Read the model definition and answer for the solid it produces. Units are mm, in the model's axes. A direction names the side the tool comes from. Round coordinates to 2 decimals unless told otherwise and drop trailing zeros. Order: outer loops, then holes, each group sorted by start corner. A loop starts at its lowest first (then second) coordinate and runs counter-clockwise, first axis right, second up. Notation, with made-up numbers: (33.5, 41) - (40.5, 41) arc R23 cw to (40.5, 65) - close; hole circle Ø6 at (-7.5, -23). An arc over 180 degrees is marked (long way). Put each result on its own line as item: value. Start each with the question number.
Q1. Which of the six approach directions +Z, -Z, +X, -X, +Y, -Y give full straight-line access (tool end or side, diameter ignored) to faces 4 (the face through (15.875, -3, -24)), 5 (the face through (3, -6.35, -14))?
Q2. Section A-A on y = -2 is taken. State how many separate pieces and enclosed holes the cut face has, then the cut area to 3 significant figures.
Q3. Section C-C on z = -6 is taken. Give the vertices of the cut face in (x, y) (3 decimals).
Q4. For a pull along Z with two mould halves and no side action, classify faces 1 (the face through (22, -3, -62.454)), 2 (the face through (30, -3, -46.579)), 3 (the face through (-0.42, -3.13, -56.03)) as pulls with the +Z half, pulls with the -Z half, needs draft (parallel to the pull), parting line crosses it, or undercut.
Q5. Section B-B on z = -28 is taken. Give the vertices of the cut face in (x, y) (3 decimals), then the cut area to 3 significant figures.
Q6. Find the intervals of material crossed by line 1 along Z through (x, y) = (2, -2.75); line 2 along Z through (x, y) = (-2, -2.5); line 3 along Z through (x, y) = (21, -2), in increasing order. Write a range as from..to.
Q7. Each of these flat-tipped pins is pushed along its axis until it touches: pin 1 Ø7.5 at (x, z) = (0.27, -52.93) entering from +Y; pin 2 Ø1 at (y, z) = (-4, -41) entering from +X (3 decimals); pin 3 Ø1.9 at (x, y) = (31, -3.5) entering from +Z; pin 4 Ø5 at (x, z) = (0, 0) entering from -Y. Where does it stop, or does it pass through?
from build123d import *

# Parameters (mm, degrees)
F0_R     = 3.175
F1_DEPTH = 6.35


# Not quite as in the source:
# - the program builds the solid bodies; features that only make, move or delete a surface that nothing else refers to are left out


with BuildPart() as f1:
    # F0 (on Front) → F1 (new body)
    with BuildSketch(Plane.XZ):
        with BuildLine():
            ThreePointArc((15.7504882737, 1.984375), (10.5003255158, 11.90625), (0, 15.875))
            ThreePointArc((0, 15.875), (-10.500325544, 11.9062499751), (-15.7504882831, 1.9843749253))
            ThreePointArc((-15.7504882831, 1.9843749253), (-15.875, -5.44e-08), (-15.7504882695, -1.9843750333))
            ThreePointArc((-15.7504882695, -1.9843750333), (0.9941387534, -15.8438414893), (15.875, 0))
            ThreePointArc((15.875, 0), (15.8440389276, 0.9909871135), (15.7512764776, 1.9781087752))
            ThreePointArc((15.7512764776, 1.9781087752), (15.7508826872, 1.9812419268), (15.7504882737, 1.984375))
        make_face()
        with BuildLine():
            ThreePointArc((0, 3.175), (2.2450640303, 2.2450640303), (3.175, 0))
            ThreePointArc((3.175, 0), (-2.2450640303, -2.2450640303), (0, 3.175))
        make_face(mode=Mode.SUBTRACT)
        with BuildLine():
            ThreePointArc((-15.7504882831, 1.9843749253), (-10.500325544, 11.9062499751), (0, 15.875))
            Line((0, 15.875), (0, 41.275))
            ThreePointArc((0, 41.275), (-7.14375, 44.4998046905), (-9.4502929642, 51.990625))
            Line((-9.4502929642, 51.990625), (-15.7504882831, 1.9843749253))
        make_face()
        with BuildLine():
            Line((0, 41.275), (0, 15.875))
            ThreePointArc((0, 15.875), (10.5003255158, 11.90625), (15.7504882737, 1.984375))
            Line((15.7504882737, 1.984375), (9.4502929642, 51.990625))
            ThreePointArc((9.4502929642, 51.990625), (9.5063048942, 51.396483242), (9.525, 50.8))
            ThreePointArc((9.525, 50.8), (6.7351920908, 44.0648079092), (0, 41.275))
        make_face()
        with BuildLine():
            ThreePointArc((-15.7504882695, -1.9843750333), (-15.875, -5.44e-08), (-15.7504882831, 1.9843749253))
            Line((-15.7504882831, 1.9843749253), (-16.0004960241, 0))
            Line((-16.0004960241, 0), (-15.7504882695, -1.9843750333))
        make_face()
        with BuildLine():
            ThreePointArc((-9.4502929642, 51.990625), (-7.14375, 44.4998046905), (0, 41.275))
            ThreePointArc((0, 41.275), (6.7351920908, 44.0648079092), (9.525, 50.8))
            ThreePointArc((9.525, 50.8), (9.5063048942, 51.396483242), (9.4502929642, 51.990625))
            ThreePointArc((9.4502929642, 51.990625), (0, 60.325), (-9.4502929642, 51.990625))
        make_face()
        with BuildLine():
            ThreePointArc((3.175, 50.8), (2.2450640303, 48.5549359697), (0, 47.625))
            ThreePointArc((0, 47.625), (-2.2450640303, 53.0450640303), (3.175, 50.8))
        make_face(mode=Mode.SUBTRACT)
        with BuildLine():
            ThreePointArc((15.875, 0), (0.9941387534, -15.8438414893), (-15.7504882695, -1.9843750333))
            Line((-15.7504882695, -1.9843750333), (-9.182062028, -54.1196420534))
            ThreePointArc((-9.182062028, -54.1196420534), (-6.9635285808, -46.7300430021), (0, -43.4077945917))
            ThreePointArc((0, -43.4077945917), (0.9024529842, -43.4251553439), (1.7992106078, -43.5278614731))
            ThreePointArc((1.7992106078, -43.5278614731), (7.5245456473, -46.7588045924), (9.7932309362, -52.9290170534))
            ThreePointArc((9.7932309362, -52.9290170534), (7.003423027, -59.6642091442), (0.2682309362, -62.4540170534))
            Line((0.2682309362, -62.4540170534), (44.7182309362, -62.4540170534))
            ThreePointArc((44.7182309362, -62.4540170534), (36.7807309362, -54.5165170534), (44.7182309362, -46.5790170534))
            Line((44.7182309362, -46.5790170534), (15.875, -46.5790170534))
            Line((15.875, -46.5790170534), (15.875, 0))
        make_face()
        with BuildLine():
            ThreePointArc((0, -43.4077945917), (-6.9635285808, -46.7300430021), (-9.182062028, -54.1196420534))
            ThreePointArc((-9.182062028, -54.1196420534), (-6.0319643733, -60.0727670534), (0.2682309362, -62.4540170534))
            ThreePointArc((0.2682309362, -62.4540170534), (7.003423027, -59.6642091442), (9.7932309362, -52.9290170534))
            ThreePointArc((9.7932309362, -52.9290170534), (7.5245456473, -46.7588045924), (1.7992106078, -43.5278614731))
            Line((1.7992106078, -43.5278614731), (0, -43.4077945917))
        make_face()
        with Locations((0.2682309362, -52.9290170534)):
            Circle(F0_R, mode=Mode.SUBTRACT)
        with BuildLine():
            ThreePointArc((52.6557309362, -54.5165170534), (50.3308910119, -48.9038569777), (44.7182309362, -46.5790170534))
            ThreePointArc((44.7182309362, -46.5790170534), (36.7807309362, -54.5165170534), (44.7182309362, -62.4540170534))
            ThreePointArc((44.7182309362, -62.4540170534), (50.3308910119, -60.1291771291), (52.6557309362, -54.5165170534))
        make_face()
        with Locations((44.7182309362, -54.5165170534)):
            Circle(F0_R, mode=Mode.SUBTRACT)
    extrude(amount=F1_DEPTH)


solid = f1.part
Findings:
1. face 4: +Z, +X, +Y, -Y
1. face 5: +Z, -Z, +X, -X, -Y
2. separate pieces: 1
2. enclosed holes: 5
2. area: 3,600 mm2
3. outline: (-15.245, -6.35) - (15.875, -6.35) - (15.875, 0) - (-15.245, 0) - close
4. face 1: pulls with the -Z half
4. face 2: pulls with the +Z half
4. face 3: undercut
5. outline: (-12.473, -6.35) - (15.875, -6.35) - (15.875, 0) - (-12.473, 0) - close
5. area: 180 mm2
6. line 1: -62.45..-55.59, -50.27..-2.47, 2.47..48.33, 53.27..60.11
6. line 2: -62.18..-55.15, -50.71..-2.47, 2.47..48.33, 53.27..60.11
6. line 3: -62.45..-46.58
7. pin 1: y = 0
7. pin 2: x = 15.875
7. pin 3: z = -46.58
7. pin 4: through
